```python
from build123d import *

# Parameters (mm, degrees)
SKETCH018_R      = 1.955414
SKETCH018_R_2    = 1.945
SKETCH018_R_3    = 1.945712
EXTRUDE021_DEPTH = 30
SKETCH017_R      = 2.552893
SKETCH017_R_2    = 2.443798
EXTRUDE020_DEPTH = 10
SKETCH003_R      = 2.9
EXTRUDE004_DEPTH = 50
EXTRUDE001_DEPTH = 10


with BuildPart() as extrude021:
    # Sketch018 (on Face20 of Fusion002) → Extrude021 (new body)
    with BuildSketch(Plane.XY.offset(36)):
        with Locations((74.789169, 44.062363)):
            Circle(SKETCH018_R)
        with Locations((111.023758, 44.110783)):
            Circle(SKETCH018_R)
        with Locations((29.159777, 78.682182)):
            Circle(SKETCH018_R_2)
        with Locations((60.039303, 78.850616)):
            Circle(SKETCH018_R_3)
        with Locations((64.412148, 25.488655)):
            Circle(SKETCH018_R_3)
    extrude(amount=EXTRUDE021_DEPTH)


with BuildPart() as extrude021_1:
    # Extrude021 placement: moved
    add(extrude021.part.moved(Location((0, 0, -22))))


with BuildPart() as base_tornillos:
    # Sketch017 (on Face5 of Cut001) → Extrude020 (new body)
    with BuildSketch(Plane.XY.offset(30)):
        with Locations((74.792107, 44.0089)):
            Circle(SKETCH017_R)
        with Locations((111.059273, 44.092655)):
            Circle(SKETCH017_R)
        with Locations((60.050713, 78.85218)):
            Circle(SKETCH017_R_2)
        with Locations((29.144051, 78.600906)):
            Circle(SKETCH017_R_2)
        with Locations((14.570175, 25.247131)):
            Circle(SKETCH017_R_2)
        with Locations((64.40612, 25.414646)):
            Circle(SKETCH017_R_2)
    extrude(amount=EXTRUDE020_DEPTH)


with BuildPart() as base_tornillos_1:
    # Extrude020 placement: moved
    add(base_tornillos.part.moved(Location((0, 0, -4))))


with BuildPart() as tornillos001:
    # Sketch003 (on Face8 of Extrude002) → Extrude004 (new body)
    with BuildSketch(Plane.XY.offset(10)):
        with Locations((10, 80.016689)):
            Circle(SKETCH003_R)
        with Locations((10, 45.008344)):
            Circle(SKETCH003_R)
        with Locations((10, 10)):
            Circle(SKETCH003_R)
    extrude(amount=EXTRUDE004_DEPTH)


with BuildPart() as tornillos001_1:
    # Extrude004 placement: moved
    add(tornillos001.part.moved(Location((0, 0, -21))))


with BuildPart() as obj1:
    # Sketch001 → Extrude001 (new body)
    with BuildSketch(Plane.XY):
        Polygon((0, 0), (30, 0), (120, 10), (120, 80), (30, 90), (0, 90), align=None)
    extrude(amount=EXTRUDE001_DEPTH)

    # Cut001: cut Tornillos001
    add(tornillos001_1.part, mode=Mode.SUBTRACT)


with BuildPart() as obj1_1:
    # Cut001 placement: moved
    add(obj1.part.moved(Location((0, 0, 20))))

    # Fusion002: union Base tornillos
    add(base_tornillos_1.part)

    # Cut009: cut Extrude021
    add(extrude021_1.part, mode=Mode.SUBTRACT)


solid = obj1_1.part
```
For this review, take the finished solid that the model builds, in its own axes (mm). A direction names the side the tool comes from. Round coordinates to 2 decimals unless told otherwise and drop trailing zeros. Write each loop counter-clockwise with the first axis right and the second up, starting at its lowest first coordinate (ties: lowest second). Pieces come first, ordered by that corner, then holes. Notation, with made-up numbers: (41.5, -33) -> (87.5, -33) arc R31 ccw to (87.5, -2) -> close; hole circle Ø8 at (44.5, 34). An arc over 180 degrees is marked (long way). One line per question, with ' | ' between items. Start each with the question number.
1) For pin 1 Ø4 at (x, y) = (87.5, 21) entering from +Z; pin 2 Ø8 at (x, z) = (86, 28.5) entering from -Y, all flat-tipped, find the tip position at first contact; note any pin that passes through.
2) Add section D-D (x = 41.5). Write out the cut boundary in (y, z).
3) Mouldability with a two-part tool opening along X and no side actions: class faces 1 (the flat face through (76, 42, 36)), 2 (the flat face through (74.37, 4.93, 24.93)), 3 (the cylindrical face through (112.24, 41.83, 32.96)), 4 (the cylindrical face through (9.371, 42.177, 24.93)) as +X half, -X half, draft (parallel to the pull), parting line (faces both ways), or undercut.
4) Add section C-C (y = 60). Write out the cut boundary in (x, z), and give its area (3 significant figures).
5) Add section B-B (z = 31.5). Count the separate pieces of the cut face and the enclosed holes in it, and give its area (3 significant figures).
6) Add section A-A (x = 10). Write out the cut boundary in (y, z).
7) Machinability: for faces 5 (the cylindrical face through (58.11, 77.37, 32.96)), 6 (the cylindrical face through (74.365, 42.153, 27.888)), which of the approach directions +Z, -Z, +X, -X, +Y, -Y give a long, thin tool a straight path to every point of the face, cutting with its end or side? Answer none if there is none.
8) Wall thickness on line 1 along Y through (x, z) = (10, 25.75); line 2 along Z through (x, y) = (82, 54); line 3 along Y through (x, z) = (66, 24.25): over which ranges is each line inside the solid? List them lowest first.
Reported:
1) pin 1: stops at z = 30 | pin 2: stops at y = 5.78
2) outline: (1.28, 20) -> (88.72, 20) -> (88.72, 30) -> (1.28, 30) -> close
3) face 1: draft | face 2: +X half | face 3: undercut | face 4: undercut
4) outline: (0, 20) -> (120, 20) -> (120, 30) -> (0, 30) -> close | area: 1,200 mm²
5) separate pieces: 6 | enclosed holes: 5 | area: 56.3 mm²
6) outline: (0, 20) -> (7.1, 20) -> (7.1, 30) -> (0, 30) -> close; (12.9, 20) -> (42.11, 20) -> (42.11, 30) -> (12.9, 30) -> close; (47.91, 20) -> (77.12, 20) -> (77.12, 30) -> (47.91, 30) -> close; (82.92, 20) -> (90, 20) -> (90, 30) -> (82.92, 30) -> close
7) face 5: +Z | face 6: +Z, -Z
8) line 1: y = 0 to 7.1, 12.9 to 42.11, 47.91 to 77.12, 82.92 to 90 | line 2: z = 20 to 30 | line 3: y = 4 to 24.36, 26.61 to 86
